```python
from build123d import *

# Parameters (mm, degrees)
F3_DEPTH = 1.27


with BuildPart() as f1:
    # F0 (on Front) → F1 (revolve)
    with BuildSketch(Plane.XZ):
        with BuildLine():
            Line((0, 0), (0, 12.5))
            ThreePointArc((0, 12.5), (-4.584632, 8.918143), (-2.218366, 3.603133))
            ThreePointArc((-2.218366, 3.603133), (-2.000063, 3.246878), (-2.20581, 2.883226))
            Line((-2.20581, 2.883226), (-5, 1.27))
            Line((-5, 1.27), (-5, 0))
            Line((-5, 0), (-1.5, 0))
            Line((-1.5, 0), (-1.5, -10))
            Line((-1.5, -10), (0, -10))
            Line((0, -10), (0, 0))
        make_face()
    revolve(axis=Axis((0, 0, 0.226223), (0, 0, -1)))

    # F2 (on Top) → F3 (join)
    with BuildSketch(Plane.XY):
        Polygon((5, -2.886751), (5, 2.886751), (0, 5.773503), (-5, 2.886751), (-5, -2.886751), (0, -5.773503), align=None)
    extrude(amount=F3_DEPTH)


solid = f1.part
```
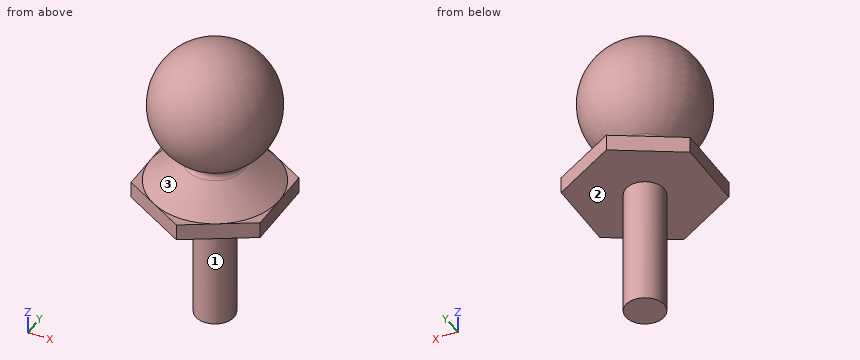
CAD build for the part. Positions are in the model's coordinates, mm. Face numbers are marked on the shaded views. Round coordinates to 2 decimals unless told otherwise and drop trailing zeros. Order: outer loops, then holes, each group sorted by start corner. A loop starts at its lowest first (then second) coordinate and runs counter-clockwise, first axis right, second up. Notation, with made-up numbers: (43, 85.25) -> (53, 85.25) arc R22 ccw to (53, 115.25) -> close; hole circle Ø6 at (-4.5, 33.5). An arc over 180 degrees is marked (long way). Write item = value, one per line.
(1) Flat gauge pins, fed straight in: P1, Ø2, axis at x = -4, y = 1.5, coming from the +Z side; P2, Ø2.5, axis at x = 4.5, y = 2, coming from the +Z side; P3, Ø2, axis at x = -4, y = -3, coming from the +Z side. Where does each tip first touch, or does it go through?
Answers follow:
P1 = 11.18
P2 = 10.75
P3 = 10.29
(2) Drill centre lines: L1, parallel to Z at x = 1.25, y = 2.75; L2, parallel to Z at x = 2, y = 3; L3, parallel to X at y = 0.75, z = -0.75. Where is each one in solid material? Low to high.
Answers follow:
L1 = 0 to 2.41, 4.14 to 11.41
L2 = 0 to 2.08, 4.72 to 10.83
L3 = -1.3 to 1.3
(3) Cut at A-A (z = -5.25). Write the cut outline in (x, y).
Answers follow:
outline = circle Ø3 at (0, 0)
(4) Pull direction Z, two halves, no side cores. Call the marked faces 1, 2 and 3: +Z half, -Z half, draft (parallel to the pull), parting line (faces both ways), or undercut.
Answers follow:
face_1 = draft
face_2 = -Z half
face_3 = undercut
